```python
from build123d import *

# Parameters (mm, degrees)
F0_W     = 35.56
F0_H     = 101.6
F1_DEPTH = 63.5
F3_D     = 6.35
F3_DEPTH = 48.26
F3_TIP   = 1.9077324654


with BuildPart() as f1:
    # F0 (on Front) → F1 (new body)
    with BuildSketch(Plane.XZ):
        with Locations((17.78, 50.8)):
            Rectangle(F0_W, F0_H)
    extrude(amount=F1_DEPTH)

    # F3
    with Locations(Plane.XZ.offset(63.5)):
        with Locations((17.2923281789, 43.087489903), (17.2923281789, 79.351015389)):
            Hole(F3_D / 2, depth=F3_DEPTH)
            with Locations((0, 0, -(F3_DEPTH + F3_TIP / 2))):  # 118° drill point
                Cone(0, F3_D / 2, F3_TIP, mode=Mode.SUBTRACT)


solid = f1.part
```
The listing builds one solid part. Answer for the finished solid, in the listing's coordinates (mm). A direction names the side the tool comes from. Round coordinates to 2 decimals unless told otherwise and drop trailing zeros. Loops run counter-clockwise (first coordinate to the right, second up) from the corner with the lowest first, then second, coordinate; pieces in that order, holes last.
1) For faces 5 (the face through (17.981, -39.032, 39.988)), 6 (the face through (35.56, -31, 50)), determine the directions among +Z, -Z, +X, -X, +Y, -Y from which every point of the face is accessible in a straight line to the end or side of a thin tool.
Outcome:
face 5: -Y
face 6: +Z, -Z, +X, +Y, -Y
2) Consider line 1 (Z direction, x = 15, y = -18); line 2 (Z direction, x = 19.5, y = -55); line 3 (Y direction, x = 17.5, z = 77.5). Determine where each line is inside the solid, lowest interval first.
Outcome:
line 1: z = 0 to 40.89, 45.28 to 77.15, 81.55 to 101.6
line 2: z = 0 to 40.81, 45.37 to 77.07, 81.63 to 101.6
line 3: y = -14.45 to 0
3) A cutting plane is placed at A-A on y = -50.5. Determine the outline of the cut face in (x, z) (3 decimals).
Outcome:
outline: (0, 0) - (35.56, 0) - (35.56, 101.6) - (0, 101.6) - close; hole circle Ø6.35 at (17.292, 43.087); hole circle Ø6.35 at (17.292, 79.351)
4) For a pull along X with two mould halves and no side action, classify faces 1 (the face through (17.98, -39.03, 76.25)), 2 (the face through (0, -31, 50)), 3 (the face through (17.589, -13.664, 43.552)), 4 (the face through (18, -31, 101.6)) as released by +X, released by -X, zero draft, split by the parting line, or undercut.
Outcome:
face 1: undercut
face 2: released by -X
face 3: undercut
face 4: zero draft
